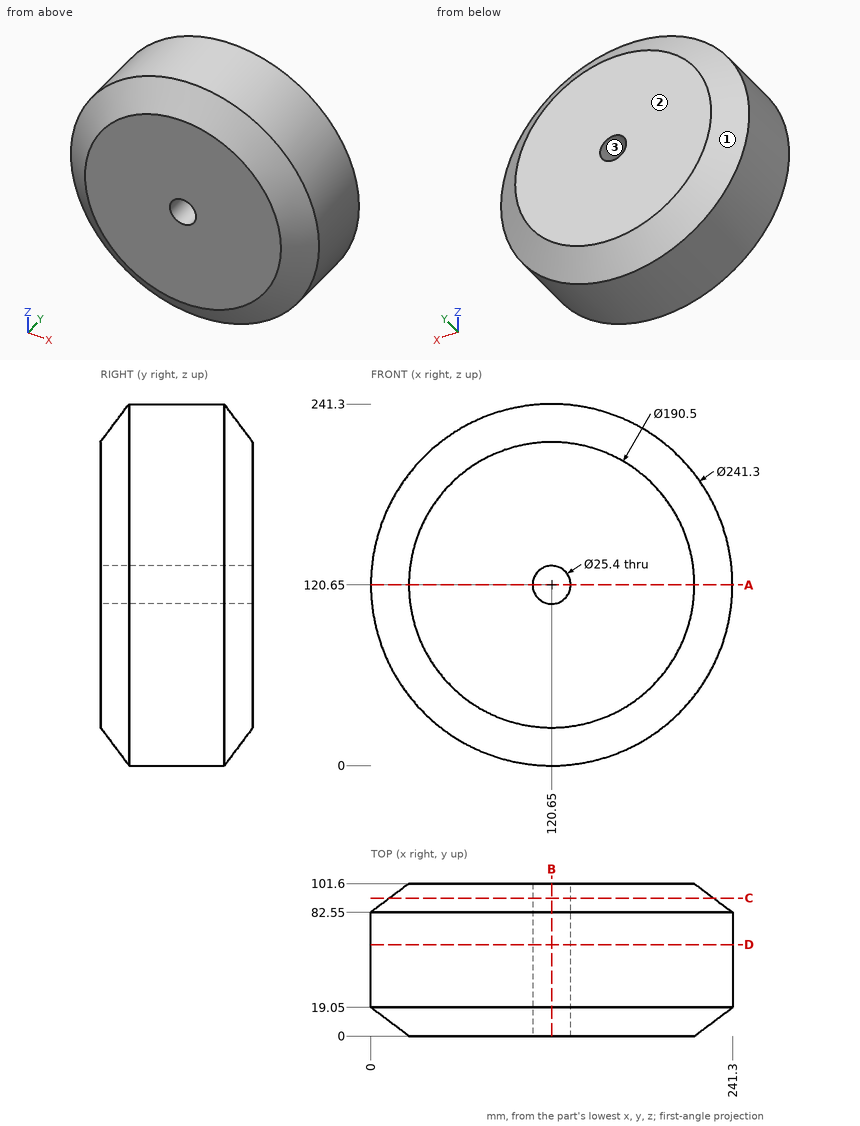
The figure shows three views and two pictorial views of one solid part (mm, origin at its lowest corner). Answer the questions. Round coordinates to 2 decimals unless told otherwise and drop trailing zeros. Write each loop counter-clockwise with the first axis right and the second up, starting at its lowest first coordinate (ties: lowest second). Pieces come first, ordered by that corner, then holes. Notation, with made-up numbers: (85, 17.5) - (133, 17.5) arc R21 ccw to (133, 32.5) - close; hole circle Ø9 at (-12.75, 35.25). An arc over 180 degrees is marked (long way). Answer in a Markdown table with one row per item. Add a question column.
1. A cutting plane is placed at B-B, the plane x = 120.65. Determine the outline of the cut face in (y, z), and give its area (3 significant figures).
2. Given pin 1 (2 mm diameter, centred on x = 70.5, y = 54, fed in from -Z); pin 2 (5 mm diameter, centred on x = 30.5, y = 29.5, fed in from +Z); pin 3 (1.5 mm diameter, centred on y = 77.5, z = 197.5, fed in from +X); pin 4 (8 mm diameter, centred on x = 145, z = 25.5, fed in from -Y), each flat-ended and moving along its own axis, determine where each tip first touches the part or whether it passes through.
3. A cutting plane is placed at C-C, the plane y = 92. Determine the outline of the cut face in (x, z).
4. A cutting plane is placed at A-A, the plane z = 120.65. Determine the outline of the cut face in (x, y).
5. Find the intervals of material crossed by line 1 along X through (y, z) = (43, 120); line 2 along Z through (x, y) = (120.65, 62.5); line 3 along X through (y, z) = (89, 126.5), in increasing order. Write a range as from..to.
6. A cutting plane is placed at D-D, the plane y = 61. Determine the outline of the cut face in (x, z), and give its area (3 significant figures).
7. The mould has two halves that part along Z. Classify the marked faces 1, 2 and 3: +Z half, -Z half, draft (parallel to the pull), parting line (faces both ways), or undercut.
Worked out:
| question | item | result |
|---|---|---|
| 1 | outline | (0, 25.4) - (19.05, 0) - (82.55, 0) - (101.6, 25.4) - (101.6, 107.95) - (0, 107.95) - close; (0, 133.35) - (101.6, 133.35) - (101.6, 215.9) - (82.55, 241.3) - (19.05, 241.3) - (0, 215.9) - close |
| 1 | area | 21,000 mm^2 |
| 2 | pin 1 | z = 10.47 |
| 2 | pin 2 | z = 203.56 |
| 2 | pin 3 | x = 214.27 |
| 2 | pin 4 | y = 0 |
| 3 | outline | circle Ø216.1 at (120.65, 120.65); hole circle Ø25.4 at (120.65, 120.65) |
| 4 | outline | (0, 19.05) - (25.4, 0) - (107.95, 0) - (107.95, 101.6) - (25.4, 101.6) - (0, 82.55) - close; (133.35, 0) - (215.9, 0) - (241.3, 19.05) - (241.3, 82.55) - (215.9, 101.6) - (133.35, 101.6) - close |
| 5 | line 1 | 0..107.97, 133.33..241.3 |
| 5 | line 2 | 0..107.95, 133.35..241.3 |
| 5 | line 3 | 8.75..109.38, 131.92..232.55 |
| 6 | outline | circle Ø241.3 at (120.65, 120.65); hole circle Ø25.4 at (120.65, 120.65) |
| 6 | area | 45,200 mm^2 |
| 7 | face 1 | parting line |
| 7 | face 2 | draft |
| 7 | face 3 | undercut |
